Verification items for the finished model (mm, model axes). Round coordinates to 2 decimals unless told otherwise and drop trailing zeros. Order: outer loops, then holes, each group sorted by start corner. A loop starts at its lowest first (then second) coordinate and runs counter-clockwise, first axis right, second up. Notation, with made-up numbers: (77.5, -19) -> (116.5, -19) arc R27 cw to (116.5, 13) -> close; hole circle Ø8 at (27.25, 44). An arc over 180 degrees is marked (long way). Return JSON: item names as keys, results as strings. Group by question number.
1) Section check A-A on z = 0. Enter the section's corners in (x, y).
2) Section check C-C on x = 1. Enter the section's corners in (y, z).
3) Section check B-B on y = 35. Enter the section's corners in (x, z).
4) Draft check along Y on faces 1 (the flat face through (2, -40, 0)), 2 (the flat face through (4, 1, 0)), 3 (the flat face through (2, 39, 3)), 4 (the cylindrical face through (1.972, -36.464, 0.325)). Enter one of: pulls with the +Y half, pulls with the -Y half, needs draft (parallel to the pull), parting line crosses it, or undercut.
5) Scan lines: L1, parallel to Y at x = 2.75, z = 0; L2, parallel to Y at x = 1, z = -0.5; L3, parallel to Y at x = 3.5, z = 3. Record each from-to range of solid material in increasing order.
```python
from build123d import *

# Parameters (mm, degrees)
SKETCH1_W           = 8
SKETCH1_H           = 80
SKETCH1_R           = 1.5
BOSS_EXTRUDE1_DEPTH = 4
CHAMFER1_SIZE       = 2


with BuildPart() as part:
    # Sketch1 → Boss-Extrude1 (new body)
    with BuildSketch(Plane(origin=(0, 0, 0), x_dir=(0, 0, -1), z_dir=(1, 0, 0))):
        Rectangle(SKETCH1_W, SKETCH1_H)
        with Locations((0, -35)):
            Circle(SKETCH1_R, mode=Mode.SUBTRACT)
        with Locations((0, 35)):
            Circle(SKETCH1_R, mode=Mode.SUBTRACT)
    extrude(amount=BOSS_EXTRUDE1_DEPTH)

    # Chamfer1
    chamfer1_edges = [part.edges().sort_by_distance(p)[0] for p in [
        (2, -40, -4),
        (2, -40, 4),
        (2, 40, 4),
        (2, 40, -4),
    ]]
    chamfer(chamfer1_edges, length=CHAMFER1_SIZE)


solid = part.part
```
Check result:
{
 "1": {"outline": "(0, -40) -> (4, -40) -> (4, -36.5) -> (0, -36.5) -> close; (0, -33.5) -> (4, -33.5) -> (4, 33.5) -> (0, 33.5) -> close; (0, 36.5) -> (4, 36.5) -> (4, 40) -> (0, 40) -> close"},
 "2": {"outline": "(-40, -2) -> (-38, -4) -> (38, -4) -> (40, -2) -> (40, 2) -> (38, 4) -> (-38, 4) -> (-40, 2) -> close; hole circle Ø3 at (-35, 0); hole circle Ø3 at (35, 0)"},
 "3": {"outline": "(0, -4) -> (4, -4) -> (4, -1.5) -> (0, -1.5) -> close; (0, 1.5) -> (4, 1.5) -> (4, 4) -> (0, 4) -> close"},
 "4": {"face 1": "pulls with the -Y half", "face 2": "needs draft", "face 3": "pulls with the +Y half", "face 4": "undercut"},
 "5": {"L1": "-40 to -36.5, -33.5 to 33.5, 36.5 to 40", "L2": "-40 to -36.41, -33.59 to 33.59, 36.41 to 40", "L3": "-39 to 39"}
}
